```python
from build123d import *

# Parameters (mm, degrees)
SKETCH2_R              = 14.2875
SKETCH2_W              = 81.28
SKETCH2_H              = 3.175
BOSS_EXTRUDE1_DEPTH    = 3.175
SKETCH9_R              = 14.2875
CUT_EXTRUDE2_DEPTH     = 3.175
BOSS_EXTRUDE2_START    = 3.175
SKETCH2_3_W            = 81.28
SKETCH2_3_H            = 3.175
BOSS_EXTRUDE2_DEPTH    = 60.7695
BOSS_EXTRUDE3_DEPTH    = 3.175
FILLET1_R              = 2.54
FILLET2_R              = 42.2275
CONVERT_SOLID2_START   = -100.6475
CONVERT_SOLID2_DEPTH   = 181.9275
CONVERT_SOLID2_2_DEPTH = 81.28


# Read off the part's stored shape, not the designer's step: Convert-Solid2
with BuildPart() as part:
    # Sketch2 → Boss-Extrude1 (new body)
    # profile 1 of 2: a face of its own
    with BuildSketch(Plane(origin=(0, 0, 0), x_dir=(0, 0, -1), z_dir=(1, 0, 0))):
        with BuildLine():
            Line((0, 3.175), (0, 69.85))
            Line((0, 69.85), (89.183866464, 160.063269699))
            ThreePointArc((89.183866464, 160.063269699), (97.582743975, 203.257963311), (60.96, 227.65258))
            Line((60.96, 227.65258), (-81.28, 227.65258))
            Line((-81.28, 227.65258), (-81.28, 69.85))
            Line((-81.28, 69.85), (-81.28, 3.175))
            Line((-81.28, 3.175), (0, 3.175))
        make_face()
        with Locations((60.96, 187.96508)):
            Circle(SKETCH2_R, mode=Mode.SUBTRACT)
    # profile 2 of 2: a face of its own
    with BuildSketch(Plane(origin=(0, 0, 0), x_dir=(0, 0, -1), z_dir=(1, 0, 0))):
        with Locations((-40.64, 1.5875)):
            Rectangle(SKETCH2_W, SKETCH2_H)
    extrude(amount=BOSS_EXTRUDE1_DEPTH)

    # Sketch9 → Cut-Extrude2 (cut)
    with BuildSketch(Plane(origin=(0, 0, 0), x_dir=(0, 0, -1), z_dir=(1, 0, 0))):
        with Locations((-49.5046, 74.46228868)):
            Circle(SKETCH9_R)
    extrude(amount=CUT_EXTRUDE2_DEPTH, mode=Mode.SUBTRACT)

    # Sketch2<3> → Boss-Extrude2 (add)
    with BuildSketch(Plane(origin=(0, 0, 0), x_dir=(0, 0, -1), z_dir=(1, 0, 0)).offset(BOSS_EXTRUDE2_START)):
        with Locations((-40.64, 1.5875)):
            Rectangle(SKETCH2_3_W, SKETCH2_3_H)
    extrude(amount=BOSS_EXTRUDE2_DEPTH)

    # Sketch3 → Boss-Extrude3 (add)
    with BuildSketch(Plane(origin=(0, 3.175, 0), x_dir=(1, 0, 0), z_dir=(0, 1, 0))):
        Polygon((63.9445, 0), (63.9445, 56.3245), (7.62, 0), align=None)
    extrude(amount=-BOSS_EXTRUDE3_DEPTH)

    # Fillet1
    fillet1_edges = [part.edges().sort_by_distance(p)[0] for p in [
        (63.9445, 1.5875, 81.28),
        (63.9445, 1.5875, -56.3245),
    ]]
    fillet(fillet1_edges, radius=FILLET1_R)

    # Fillet2
    fillet2_edges = [part.edges().sort_by_distance(p)[0] for p in [
        (1.5875, 227.65258, 81.28),
    ]]
    fillet(fillet2_edges, radius=FILLET2_R)

    # Convert-Solid2 outline → Convert-Solid2 (cut)
    with BuildSketch(Plane.XY.offset(CONVERT_SOLID2_START)):
        with BuildLine():
            Line((0, 0), (6.21284, 0))
            ThreePointArc((6.21284, 0), (1.819698706, 1.819698706), (0, 6.21284))
            Line((0, 6.21284), (0, 0))
        make_face()
        with BuildLine():
            Line((6.21284, 3.03784), (63.9445, 3.03784))
            Line((63.9445, 3.03784), (63.9445, 3.175))
            Line((63.9445, 3.175), (5.289718593, 3.175))
            ThreePointArc((5.289718593, 3.175), (5.746212204, 3.072317193), (6.21284, 3.03784))
        make_face()
        with BuildLine():
            Line((3.175, 227.65258), (3.03784, 227.65258))
            Line((3.03784, 227.65258), (3.03784, 6.21284))
            ThreePointArc((3.03784, 6.21284), (3.072317193, 5.746212204), (3.175, 5.289718593))
            Line((3.175, 5.289718593), (3.175, 227.65258))
        make_face()
    extrude(amount=CONVERT_SOLID2_DEPTH, mode=Mode.SUBTRACT)

    # Convert-Solid2 2 outline → Convert-Solid2 2 (add)
    with BuildSketch(Plane.XY):
        with BuildLine():
            Line((3.175, 3.175), (5.289718593, 3.175))
            ThreePointArc((5.289718593, 3.175), (3.96777597, 3.96777597), (3.175, 5.289718593))
            Line((3.175, 5.289718593), (3.175, 3.175))
        make_face()
    extrude(amount=CONVERT_SOLID2_2_DEPTH)


solid = part.part
```
Geometry: final body of the model. Coordinates: model frame, mm. A direction names the side the tool comes from. Coordinates: 2 decimals unless noted, no trailing zeros. Order: outer loops, then holes, each group sorted by start corner. A loop starts at its lowest first (then second) coordinate and runs counter-clockwise, first axis right, second up. Notation, with made-up numbers: (10, 59) -> (60, 59) arc R22 ccw to (60, 68) -> close; hole circle Ø4 at (68.5, 5.5). An arc over 180 degrees is marked (long way). Write each question's results on one line, items separated by ' | '. Start each with the question number.
1) Cut plane A-A, the plane y = 78. Output: boundary loops of the cut face in (x, z).
2) Cut plane D-D, the plane x = 13.5. Output: boundary loops of the cut face in (y, z).
3) Material intervals for line 1 along X through (y, z) = (83, -9.5); line 2 along Y through (x, z) = (1, -60), sorted ascending.
4) Mould query, pull axis Y, two halves, no side actions, for faces 3 (the flat face through (35, 3.038, 28)), 4 (the flat face through (35, 0, 28)), 5 (the cylindrical face through (1.5, 179.3, -49.6)). Classes: released by +Y, released by -Y, zero draft, split by the parting line, or undercut.
5) Set-up query: faces 1 (the flat face through (3.038, 143, 9)), 2 (the flat face through (33.98, 1.54, -26.36)). Return all of +Z, -Z, +X, -X, +Y, -Y with unobstructed straight access to the full face (end or side cutting, diameter ignored); none if empty.
6) First-contact query: pin 1 (5 mm diameter, centred on y = 118.5, z = -12.5, fed in from +X); pin 2 (10 mm diameter, centred on x = 26.5, z = -21.5, fed in from -Y); pin 3 (6 mm diameter, centred on x = 5, y = 21, fed in from -Z); pin 4 (12 mm diameter, centred on x = 9.5, z = 26.5, fed in from +Y). Flat tips, straight axial feed; report the tip coordinate or a pass-through.
Checks:
1) outline: (0, -8.06) -> (3.04, -8.06) -> (3.04, 35.66) -> (0, 35.66) -> close; (0, 63.35) -> (3.04, 63.35) -> (3.04, 81.28) -> (0, 81.28) -> close
2) outline: (0, -5.88) -> (3.04, -5.88) -> (3.04, 81.28) -> (0, 81.28) -> close
3) line 1: 0 to 3.04 | line 2: 130.54 to 173.71, 202.22 to 227.65
4) face 3: released by +Y | face 4: released by -Y | face 5: undercut
5) face 1: +Z, -Z, +X, +Y | face 2: -Z, -X, +Y, -Y
6) pin 1: x = 3.04 | pin 2: y = 0 | pin 3: z = 0 | pin 4: y = 4.56
